The listing builds one solid part. Answer for the finished solid, in the listing's coordinates (mm). A direction names the side the tool comes from. Round coordinates to 2 decimals unless told otherwise and drop trailing zeros. Loops run counter-clockwise (first coordinate to the right, second up) from the corner with the lowest first, then second, coordinate; pieces in that order, holes last. Notation, with made-up numbers: M 22,-7.75 L 59,-7.75 A21 ccw 59,12.25 Z; hole C 60,82 d4. An arc over 180 degrees is marked long. Answer as a JSON object with one key per item and string values.
```python
from build123d import *

# Parameters (mm, degrees)
BOSS_EXTRU_1_DEPTH      = 27
CONG_1_R                = 5
ESQUISSE2_R             = 2.25
ENL_V_MAT_EXTRU_1_DEPTH = 44.943145085
ENL_V_MAT_EXTRU_2_DEPTH = 27
CONG_2_R                = 3
ESQUISSE4_R             = 2
ENL_V_MAT_EXTRU_3_DEPTH = 37.908671068


with BuildPart() as part:
    # Esquisse1 → Boss.-Extru.1 (new body)
    with BuildSketch(Plane.XY):
        Polygon((0, 0), (29, 0), (29, 2), (16.5, 2), (16.5, 19), (12.5, 19), (12.5, 2), (0, 2), align=None)
    extrude(amount=BOSS_EXTRU_1_DEPTH)

    # Congé1
    cong_1_edges = [part.edges().sort_by_distance(p)[0] for p in [
        (29, 1, 27),
        (0, 1, 0),
        (0, 1, 27),
        (29, 1, 0),
    ]]
    fillet(cong_1_edges, radius=CONG_1_R)

    # Esquisse2 → Enlèv. mat.-Extru.1 (cut, through all)
    with BuildSketch(Plane.XZ):
        with Locations(Location((5.5, 21.5, 0), (0, 0, 270))):
            Circle(ESQUISSE2_R)
        with Locations(Location((5.5, 5.5, 0), (0, 0, 270))):
            Circle(ESQUISSE2_R)
        with Locations(Location((23.5, 5.5, 0), (0, 0, 270))):
            Circle(ESQUISSE2_R)
        with Locations(Location((23.5, 21.5, 0), (0, 0, 270))):
            Circle(ESQUISSE2_R)
    extrude(amount=-ENL_V_MAT_EXTRU_1_DEPTH, mode=Mode.SUBTRACT)

    # Esquisse3 → Enlèv. mat.-Extru.2 (cut)
    with BuildSketch(Plane.ZY.offset(-12.5)):
        with BuildLine():
            Line((0, 9), (9, 9))
            Line((9, 9), (16.629670691, 17.110987927))
            ThreePointArc((16.629670691, 17.110987927), (23.21111105, 18.577722468), (27, 13))
            Line((27, 13), (29.874608193, 13))
            Line((29.874608193, 13), (29.874608193, 22.034695391))
            Line((29.874608193, 22.034695391), (0, 22.034695391))
            Line((0, 22.034695391), (0, 9))
        make_face()
    extrude(amount=-ENL_V_MAT_EXTRU_2_DEPTH, mode=Mode.SUBTRACT)

    # Congé2
    cong_2_edges = [part.edges().sort_by_distance(p)[0] for p in [
        (14.5, 9, 0),
        (14.5, 9, 9),
    ]]
    fillet(cong_2_edges, radius=CONG_2_R)

    # Esquisse4 → Enlèv. mat.-Extru.3 (cut, through all)
    with BuildSketch(Plane.ZY.offset(-12.5)):
        with Locations((21, 13)):
            Circle(ESQUISSE4_R)
    extrude(amount=-ENL_V_MAT_EXTRU_3_DEPTH, mode=Mode.SUBTRACT)


solid = part.part
```
Item 1: Straight lines are drawn through the part: line 1 (X direction, y = 0.65, z = 21.5); line 2 (Y direction, x = 14.8, z = 21); line 3 (X direction, y = 4.5, z = 11.75). For each, find the intervals that lie inside material, in ascending order.
Values follow:
{"line 1": "0 to 3.25, 7.75 to 21.25, 25.75 to 29", "line 2": "0 to 11, 15 to 19", "line 3": "12.5 to 16.5"}
Item 2: The part is cut by section C-C (x = 4.5). Give the vertices of the cut face in (y, z).
Values follow:
{"outline": "M 0,0.03 L 2,0.03 L 2,3.48 L 0,3.48 Z; M 0,7.52 L 2,7.52 L 2,19.48 L 0,19.48 Z; M 0,23.52 L 2,23.52 L 2,26.97 L 0,26.97 Z"}
Item 3: The part is cut by section A-A (x = 13.75). Give the vertices of the cut face in (y, z), then the cut area to 3 significant figures.
Values follow:
{"outline": "M 0,0 L 6,0 A3 ccw 9,3 L 9,7.7 A3 cw 9.94,9.89 L 17.11,16.63 A6 ccw 13,27 L 0,27 Z; hole C 13,21 d4", "area": "353 mm^2"}
Item 4: Which of the six approach directions +Z, -Z, +X, -X, +Y, -Y give full straight-line access (tool end or side, diameter ignored) to faces 1 (the face through (23, 2, 13)), 2 (the face through (14, 2, 0)), 3 (the face through (0, 1, 13)), 4 (the face through (14, 9, 5)), 5 (the face through (6, 2, 13))?
Values follow:
{"face 1": "+Z, -Z, +X, +Y", "face 2": "-Z, +X, -X, +Y, -Y", "face 3": "+Z, -Z, -X, +Y, -Y", "face 4": "-Z, +X, -X, +Y", "face 5": "+Z, -Z, -X, +Y"}
Item 5: The part is cut by section B-B (y = 1.5). Give the vertices of the cut face in (x, z), then the cut area to 3 significant figures.
Values follow:
{"outline": "M 0,5 A5 ccw 5,0 L 24,0 A5 ccw 29,5 L 29,22 A5 ccw 24,27 L 5,27 A5 ccw 0,22 Z; hole C 5.5,5.5 d4.5; hole C 5.5,21.5 d4.5; hole C 23.5,5.5 d4.5; hole C 23.5,21.5 d4.5", "area": "698 mm^2"}
Item 6: The part is cut by section D-D (z = 21.5). Give the vertices of the cut face in (x, y).
Values follow:
{"outline": "M 0,0 L 3.25,0 L 3.25,2 L 0,2 Z; M 7.75,0 L 21.25,0 L 21.25,2 L 16.5,2 L 16.5,11.06 L 12.5,11.06 L 12.5,2 L 7.75,2 Z; M 12.5,14.94 L 16.5,14.94 L 16.5,18.98 L 12.5,18.98 Z; M 25.75,0 L 29,0 L 29,2 L 25.75,2 Z"}
Item 7: Flat-ended cylindrical pins translate along their axes: P1, Ø4, axis at x = 23, z = 18, coming from the +Y side; P2, Ø5, axis at y = 6.5, z = 12, coming from the +X side; P3, Ø1, axis at y = 4.5, z = 6, coming from the -X side. Find the tip coordinate at first contact, or state that the pin passes through.
Values follow:
{"P1": "y = 2", "P2": "x = 16.5", "P3": "x = 12.5"}
Item 8: Determine the mould class of faces 6 (the face through (14.53, 8.14, 0.9)), 7 (the face through (14.472, 14.352, 19.526)), 8 (the face through (14, 0, 13)), 9 (the face through (12.5, 9, 16)) for opening direction Y: released by +Y, released by -Y, zero draft, split by the parting line, or undercut.
Values follow:
{"face 6": "released by +Y", "face 7": "undercut", "face 8": "released by -Y", "face 9": "zero draft"}
